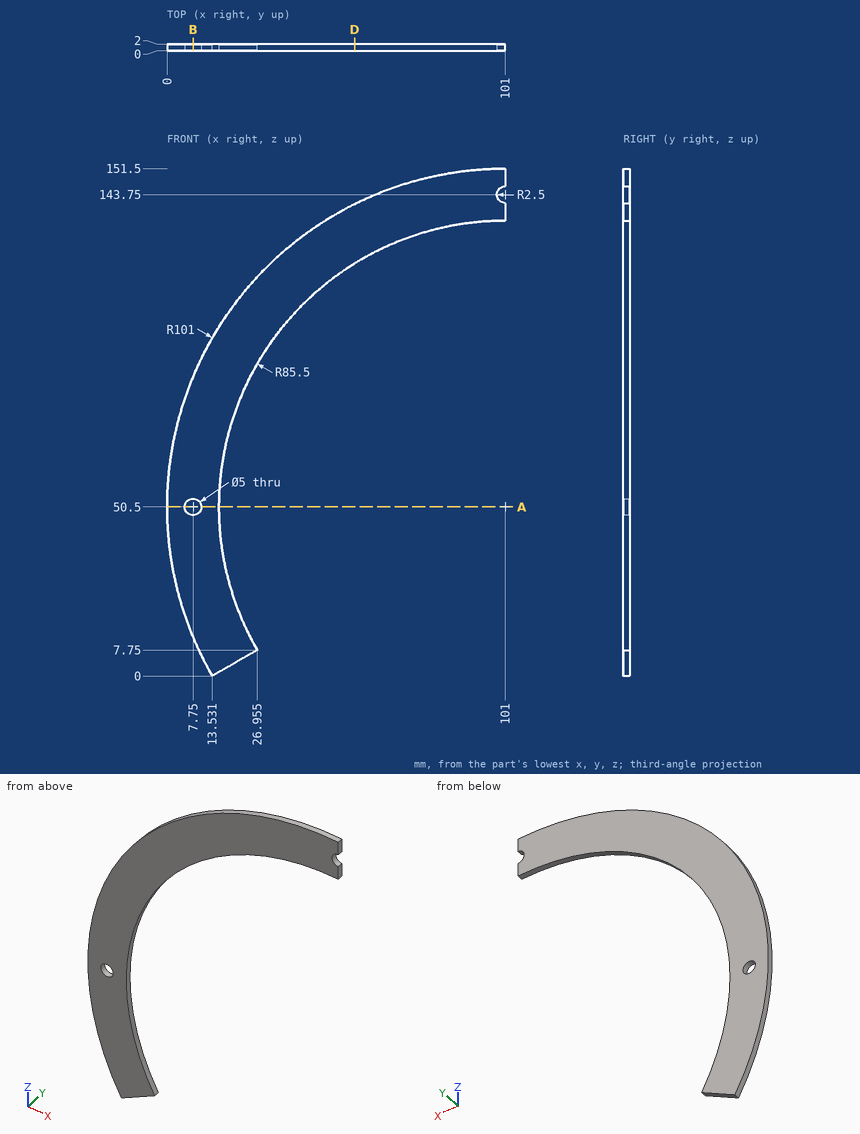
Verification items for this drawing (mm, ordinates from the low corner). Coordinates: 2 decimals unless noted, no trailing zeros. Write each loop counter-clockwise with the first axis right and the second up, starting at its lowest first coordinate (ties: lowest second). Pieces come first, ordered by that corner, then holes. Notation, with made-up numbers: M 66.25,-20 L 77.25,-20 A15 cw 77.25,0 Z; hole C 19,59.5 d1. An arc over 180 degrees is marked long. One line per item, written item: value. Start each with the question number.
(1) Sectioned sample at D-D, the plane x = 56. Enter the section's corners in (y, z).
(2) Scan lines: line 1 along X through (y, z) = (0.9, 50.5); line 2 along X through (y, z) = (0.85, 120) (1 decimal); line 3 along X through (y, z) = (1, 77.5) (1 decimal). Record each from-to range of solid material in increasing order. Write a range as [from, to].
(3) Depth check by flat-ended pin: pin 1 (2 mm diameter, centred on x = 70.5, z = 128.5, fed in from +Y). Enter the tip coordinate at first touch or a pass-through.
(4) Sectioned sample at A-A, the plane z = 50.5. Enter the section's corners in (x, y), and give its area (3 significant figures).
(5) Sectioned sample at B-B, the plane x = 7.75. Enter the section's corners in (y, z).
Filled sheet:
1. outline: M 0,123.2 L 2,123.2 L 2,140.92 L 0,140.92 Z
2. line 1: [0, 5.25], [10.25, 15.5]
2. line 2: [27.7, 51.2]
2. line 3: [3.7, 19.9]
3. pin 1: through
4. outline: M 0,0 L 5.25,0 L 5.25,2 L 0,2 Z; M 10.25,0 L 15.5,0 L 15.5,2 L 10.25,2 Z
4. area: 21.0 mm²
5. outline: M 0,11.7 L 2,11.7 L 2,48 L 0,48 Z; M 0,53 L 2,53 L 2,89.3 L 0,89.3 Z
